Can you work these out from the model? Positions are in its coordinate system, mm. Face numbers are marked on the shaded views. A direction names the side the tool comes from. Give positions to 0.01 mm unless a question says otherwise; leave off trailing zeros. Order: outer loops, then holes, each group sorted by start corner. A loop starts at its lowest first (then second) coordinate and runs counter-clockwise, first axis right, second up.
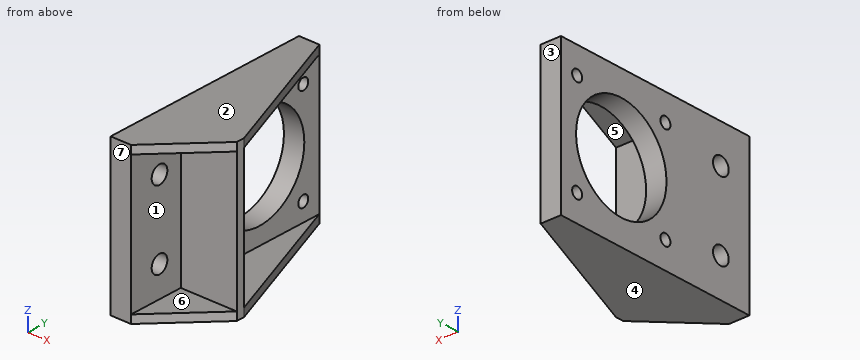
Autodesk Inventor part; units mm, degrees
ref_plane "YZ Plane" through (0, 0, 0) normal (1, 0, 0) x (0, 1, 0)
ref_plane "XZ Plane" through (0, 0, 0) normal (0, 1, 0) x (-1, 0, 0)
ref_plane "XY Plane" through (0, 0, 0) normal (0, 0, 1) x (1, 0, 0)
sketch "Sketch2" plane through (0, 0, 0) normal (1, 0, 0) x (0, 1, 0)
  line L0 (-15.5, 15.5) -> (15.5, 15.5) construction
  line L1 (15.5, 15.5) -> (15.5, -15.5) construction
  line L2 (15.5, -15.5) -> (-15.5, -15.5) construction
  line L3 (-15.5, -15.5) -> (-15.5, 15.5) construction
  line L4 (-15.5, 15.5) -> (15.5, -15.5) construction
  line L5 (15.5, 15.5) -> (-15.5, -15.5) construction
  circle A0 centre (15.5, 15.5) radius 1.75
  circle A1 centre (15.5, -15.5) radius 1.75
  circle A2 centre (-15.5, -15.5) radius 1.75
  line L6 (-21.15, 21.15) -> (21.15, 21.15) construction
  line L7 (21.15, -21.15) -> (-21.15, -21.15) construction
  line L8 (-21.15, -21.15) -> (-21.15, 21.15) construction
  line L9 (-21.15, 21.15) -> (21.15, -21.15) construction
  line L10 (21.15, 21.15) -> (-21.15, -21.15) construction
  circle A3 centre (-15.5, 15.5) radius 1.75
  line L11 (21.15, 21.15) -> (-21.15, 21.15) construction
  line L12 (-21.15, 23.69) -> (21.15, 23.69)
  line L13 (21.15, -21.15) -> (-21.15, -21.15) construction
  line L14 (-21.15, -21.15) -> (-21.15, -23.69) construction
  line L15 (-21.15, -23.69) -> (21.15, -23.69)
  line L16 (-21.15, 21.15) -> (-44.96, 21.15) construction
  line L17 (-44.96, 21.15) -> (-44.96, -21.15)
  line L18 (-44.96, -21.15) -> (-21.15, -21.15) construction
  line L19 (-21.15, -21.15) -> (-21.15, 21.15) construction
  line L20 (-44.96, 21.15) -> (-20.6909, 21.15) construction
  line L21 (-44.96, -21.15) -> (-21.15, -21.15) construction
  line L22 (-34.96, 0.6795) -> (-34.96, -24.3695) construction
  line L23 (-34.96, 0.6795) -> (-34.96, 23.0105) construction
  circle A4 centre (-34.96, 11.845) radius 2.75
  circle A5 centre (-34.96, -11.845) radius 2.75
  circle A6 centre (0, 0) radius 15.875
  line L24 (-21.15, -23.69) -> (-24.96, -23.69)
  line L25 (-24.96, -23.69) -> (-24.96, 23.69) construction
  line L26 (-24.96, 23.69) -> (-21.15, 23.69)
  line L27 (-21.15, 23.69) -> (-21.15, -23.69) construction
  line L28 (21.15, -23.69) -> (21.15, 23.69)
  line L29 (21.15, -23.69) -> (-24.96, -23.69)
  line L30 (-24.96, -23.69) -> (-24.96, 23.69)
  line L31 (-24.96, 23.69) -> (21.15, 23.69)
  line L32 (21.15, 23.69) -> (21.15, -23.69)
  line L33 (-24.96, 23.69) -> (-44.96, 23.69)
  line L34 (-44.96, 23.69) -> (-44.96, -23.69)
  line L35 (-44.96, -23.69) -> (-24.96, -23.69)
  line L36 (-24.96, -23.69) -> (-24.96, 23.69)
  dimension "d19" = 31
  dimension "d20" = 3.5
  dimension "d21" = 42.3
  dimension "d24" = 5.5
  dimension "d35" = 31.75
  dimension "d36" = 23.69
  dimension "d38" = 20
  dimension "d39" = 42.3
  dimension "d40" = 3.81
  dimension "d41" = 10
  dimension "d42" = 2.54
  dimension "d43" = 42.3
extrude "Extrusion2" add sketch "Sketch2" along normal blind 6.35
sketch "Sketch3" plane through (6.35, 0, 0) normal (1, 0, 0) x (0, 0, -1)
  line L0 (-23.69, 21.15) -> (-23.69, -41.15)
  line L1 (-21.15, -44.96) -> (21.15, -44.96)
  line L2 (-23.69, 21.15) -> (-21.15, 21.15)
  line L3 (-21.15, 21.15) -> (-21.15, -44.96)
  line L4 (-21.15, -44.96) -> (-23.69, -44.96)
  line L5 (-23.69, -44.96) -> (-23.69, 21.15)
  line L6 (23.69, -24.96) -> (23.69, 21.15)
  line L7 (23.69, 21.15) -> (21.15, 21.15)
  line L8 (21.15, 21.15) -> (21.15, -44.96)
  line L9 (21.15, -44.96) -> (23.69, -44.96)
  line L10 (23.69, -44.96) -> (23.69, 21.15)
  line L11 (23.69, -27.5) -> (-23.69, -27.5)
  line L12 (-23.69, -27.5) -> (-23.69, -24.96)
  line L13 (-23.69, -24.96) -> (23.69, -24.96)
  line L14 (23.69, -24.96) -> (23.69, -27.5)
  point P0 (0, 0)
  point P1 (23.69, -41.15)
  dimension "d27" = 2.54
  dimension "d28" = 2.54
  dimension "d29" = 2.54
  dimension "d30" = 20
extrude "Extrusion3" add sketch "Sketch3" along normal blind 17.46 contours L2 L3 L13 L0 | L13 L3 L11 L0 | L11 L3 L4 L5 L0 | L13 L8 L11 L3 | L13 L10 L11 L8 | L8 L7 L6 L13 | L11 L10 L9 L8
sketch "Sketch5" plane through (0, -44.96, 23.69) normal (0, 0, 1) x (1, 0, 0)
  line L0 (23.81, 20) -> (6.35, 20)
  line L1 (23.81, 66.11) -> (23.81, 20)
  line L2 (6.35, 66.11) -> (23.81, 66.11)
  line L3 (6.35, 20) -> (6.35, 66.11)
  line L4 (6.35, 17.46) -> (23.81, 17.46)
  line L5 (6.35, 0) -> (6.35, 17.46)
  line L6 (6.35, 0) -> (23.81, 0)
  line L7 (23.81, 17.46) -> (23.81, 0)
  line L8 (6.35, 0) -> (6.35, 17.46)
  line L9 (23.81, 17.46) -> (6.35, 0)
  line L10 (23.81, 20) -> (6.35, 66.11)
  point P0 (0, 44.96)
extrude "Extrusion5" cut sketch "Sketch5" against normal through all contours L10 L2 L1 | L7 L6 L9
properties part number "nemaMountStock"
1) If I drill on line 1 (Z direction, x = 5, y = -34.96) (3 decimals); line 2 (Z direction, x = 9.75, y = -33.5); line 3 (Y direction, x = 4.25, z = -0.5), over which ranges is the centre line in solid material (lowest first)?
2) We'd pull the mould along Z, two halves only. Please class the marked faces 1, 2, 3 and 4: +Z half, -Z half, draft (parallel to the pull), parting line (faces both ways), or undercut.
3) Which directions (+Z, -Z, +X, -X, +Y, -Y) give clear straight access to the entire face, cutting with the end or side of a thin tool? Please do the marked faces 5, 6 and 7.
4) Suppose I cut it at D-D (z = -18). Please give me the cut outline in (x, y).
5) Suppose I cut it at B-B (z = 0). Please give me the cut outline in (x, y) (3 decimals).
6) Suppose I cut it at C-C (y = -1). Please give me the cut outline in (x, z), and give its area (3 significant figures).
7) Suppose I cut it at A-A (y = -34.96). Please give me the cut outline in (x, z) (3 decimals), and give its area (3 significant figures).
8) I'm going to push flat-ended pins straight in: pin 1 Ø4 at (y, z) = (15.5, 15.5) entering from +X; pin 2 Ø3 at (x, z) = (9, -7.5) entering from +Y; pin 3 Ø5 at (x, z) = (18, 2) entering from -Y. Where does each tip first touch, or does it pass through?
Results:
1. line 1: z = -23.69 to -14.595, -9.095 to 9.095, 14.595 to 23.69
1. line 2: z = -23.69 to -21.15, 21.15 to 23.69
1. line 3: y = -44.96 to -15.87, 15.87 to 21.15
2. face 1: undercut
2. face 2: +Z half
2. face 3: draft
2. face 4: -Z half
3. face 5: +X, +Y
3. face 6: +X, -Y
3. face 7: +Z, -Z, +X, -X, -Y
4. outline: (0, -44.96) - (6.35, -44.96) - (6.35, -27.5) - (23.81, -27.5) - (23.81, -24.96) - (6.35, -24.96) - (6.35, 21.15) - (0, 21.15) - close
5. outline: (0, -44.96) - (6.35, -44.96) - (6.35, -27.5) - (23.81, -27.5) - (23.81, -24.96) - (6.35, -24.96) - (6.35, -15.875) - (0, -15.875) - close; (0, 15.875) - (6.35, 15.875) - (6.35, 21.15) - (0, 21.15) - close
6. outline: (0, -23.69) - (14.74, -23.69) - (14.74, -21.15) - (6.35, -21.15) - (6.35, -15.84) - (0, -15.84) - close; (0, 15.84) - (6.35, 15.84) - (6.35, 21.15) - (14.74, 21.15) - (14.74, 23.69) - (0, 23.69) - close
6. area: 142 mm2
7. outline: (0, -23.69) - (16.35, -23.69) - (16.35, -21.15) - (6.35, -21.15) - (6.35, -14.595) - (0, -14.595) - close; (0, -9.095) - (6.35, -9.095) - (6.35, 9.095) - (0, 9.095) - close; (0, 14.595) - (6.35, 14.595) - (6.35, 21.15) - (16.35, 21.15) - (16.35, 23.69) - (0, 23.69) - close
7. area: 282 mm2
8. pin 1: stops at x = 6.35
8. pin 2: stops at y = -24.96
8. pin 3: stops at y = -27.5
